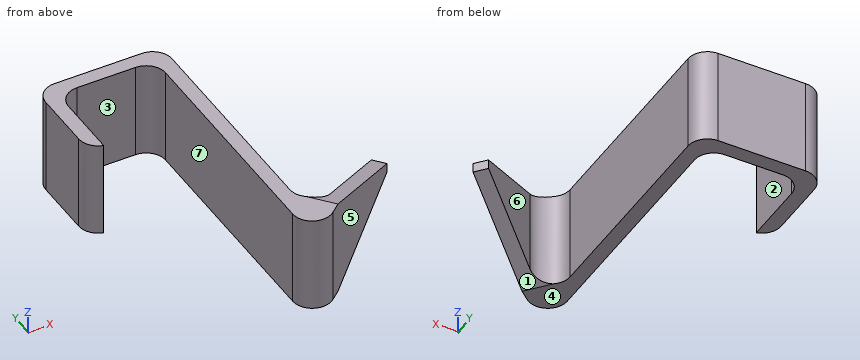
from build123d import *

# Parameters (mm, degrees)
F1_DEPTH     = 25.4
F2_T1_DEPTH  = 25.4
F2_T3_DEPTH  = 25.4
F2_T5_DEPTH  = 25.4
F2_T7_DEPTH  = 50.8
F2_T9_DEPTH  = 50.8
F2_T11_DEPTH = 49.9934442484
F3_SIZE2     = 11.4636064984
F3_SIZE      = 31.496
F3_2_SIZE2   = 11.4636064984
F3_2_SIZE    = 31.496
F4_T1_DEPTH  = 50.8
F5_T1_DEPTH  = 68.1227876391


# Not quite as in the source:
# - a fillet or chamfer that OpenCascade refuses, or shapes differently, is made with other operations: its cross-section is extruded or revolved along the edge and cut away or added


with BuildPart() as f1:
    # F0 (on Top) → F1 (new body)
    with BuildSketch(Plane.XY):
        Polygon((33.02, 0), (0, 0), (0, -25.4), (3.81, -25.4), (3.81, -3.81), (29.21, -3.81), (29.21, -76.2), (33.02, -76.2), (33.02, -71.2263982276), align=None)
        Polygon((61.7030253754, -47.1584822141), (33.02, -71.2263982276), (33.02, -76.2), (64.1520461684, -50.0771115423), align=None)
    extrude(amount=F1_DEPTH)

    # F2: fillet of radius 5.08 on 6 edges, made by hand

    # F2_s2 → F2_t1 (join)
    with BuildSketch(Plane.XY):
        with BuildLine():
            ThreePointArc((3.81, -8.89), (5.2978975516, -5.2978975516), (8.89, -3.81))
            Line((8.89, -3.81), (3.81, -3.81))
            Line((3.81, -3.81), (3.81, -8.89))
        make_face()
    extrude(amount=F2_T1_DEPTH)

    # F2_s4 → F2_t3 (join)
    with BuildSketch(Plane.XY):
        with BuildLine():
            ThreePointArc((24.13, -3.81), (27.7221024484, -5.2978975516), (29.21, -8.89))
            Line((29.21, -8.89), (29.21, -3.81))
            Line((29.21, -3.81), (24.13, -3.81))
        make_face()
    extrude(amount=F2_T3_DEPTH)

    # F2_s6 → F2_t5 (join)
    with BuildSketch(Plane.XY):
        with BuildLine():
            ThreePointArc((33.02, -60.3323030715), (35.9530992304, -64.9363466296), (41.3653610572, -64.2238088425))
            Line((41.3653610572, -64.2238088425), (33.02, -71.2263982276))
            Line((33.02, -71.2263982276), (33.02, -60.3323030715))
        make_face()
    extrude(amount=F2_T5_DEPTH)

    # F2_s8 → F2_t7 (cut)
    with BuildSketch(Plane.XY.offset(-12.7)):
        with BuildLine():
            ThreePointArc((27.94, 0), (31.5321024484, -1.4878975516), (33.02, -5.08))
            Line((33.02, -5.08), (33.02, 0))
            Line((33.02, 0), (27.94, 0))
        make_face()
    extrude(amount=F2_T7_DEPTH, mode=Mode.SUBTRACT)

    # F2_s10 → F2_t9 (cut)
    with BuildSketch(Plane.XY.offset(-12.7)):
        with BuildLine():
            ThreePointArc((5.08, 0), (1.4878975516, -1.4878975516), (0, -5.08))
            Line((0, -5.08), (0, 0))
            Line((0, 0), (5.08, 0))
        make_face()
    extrude(amount=F2_T9_DEPTH, mode=Mode.SUBTRACT)

    # F2_s12 → F2_t11 (cut)
    with BuildSketch(Plane.XY.offset(-12.2967221242)):
        with BuildLine():
            ThreePointArc((3.81, -25.4), (1.0639073716, -23.5921631237), (0, -20.4813111503))
            Line((0, -20.4813111503), (0, -25.4))
            Line((0, -25.4), (3.81, -25.4))
        make_face()
    extrude(amount=F2_T11_DEPTH, mode=Mode.SUBTRACT)

    # F3
    f3_edges = [f1.edges().sort_by_distance(p)[0] for p in [
        (62.927536, -48.617797, 25.4),
    ]]
    f3_side = f1.faces().sort_by_distance((30.827761, -2.192239, 25.4))[0]
    chamfer(f3_edges, length=F3_SIZE, length2=F3_SIZE2, reference=f3_side)

    # F3#2
    f3_2_edges = [f1.edges().sort_by_distance(p)[0] for p in [
        (62.927536, -48.617797, 0),
    ]]
    f3_2_side = f1.faces().sort_by_distance((30.827761, -2.192239, 0))[0]
    chamfer(f3_2_edges, length=F3_2_SIZE, length2=F3_2_SIZE2, reference=f3_2_side)

    # F4: fillet of radius 5.08 on 1 edges, made by hand

    # F4_s2 → F4_t1 (cut)
    with BuildSketch(Plane.XY.offset(-12.7)):
        with BuildLine():
            ThreePointArc((34.29, -76.2), (30.6978975516, -74.7121024484), (29.21, -71.12))
            Line((29.21, -71.12), (29.21, -76.2))
            Line((29.21, -76.2), (34.29, -76.2))
        make_face()
    extrude(amount=F4_T1_DEPTH, mode=Mode.SUBTRACT)

    # F5: fillet of radius 5.08 on 1 edges, made by hand

    # F5_s2 → F5_t1 (cut)
    with BuildSketch(Plane.XY.offset(-21.3613938196)):
        with BuildLine():
            ThreePointArc((37.5553610572, -72.3943802096), (32.1430992304, -73.1069179967), (29.21, -68.5028744386))
            Line((29.21, -68.5028744386), (28.702, -68.5028744386))
            ThreePointArc((28.702, -68.5028744386), (28.702, -71.12), (33.0571094194, -76.5702958467))
            Line((33.0571094194, -76.5702958467), (33.495726487, -76.4639649832))
            Line((33.495726487, -76.4639649832), (37.8818971629, -72.7835307867))
            Line((37.8818971629, -72.7835307867), (37.5553610572, -72.3943802096))
        make_face()
    extrude(amount=F5_T1_DEPTH, mode=Mode.SUBTRACT)


solid = f1.part
Design review of the part built by this model. Coordinates are the model's own, in mm. Face numbers are marked on the shaded views. A direction names the side the tool comes from. Round coordinates to 2 decimals unless told otherwise and drop trailing zeros. Order: outer loops, then holes, each group sorted by start corner. A loop starts at its lowest first (then second) coordinate and runs counter-clockwise, first axis right, second up.
1) Consider section C-C (y = -52). State the section outline as (x, z) points.
The answers:
outline: (29.21, 0) - (33.02, 0) - (33.02, 25.4) - (29.21, 25.4) - close; (55.93, 8.72) - (61.86, 10.37) - (61.86, 15.03) - (55.93, 16.68) - close
2) For L1, parallel to X at y = -20, z = 23.25; L2, parallel to X at y = -31, z = 5.5; L3, parallel to Y at x = 23, z = 15, list the stretches that pass through material, from the lowest coordinate up.
The answers:
L1: x = 0 to 3.81, 29.21 to 33.02
L2: x = 29.21 to 33.02
L3: y = -3.81 to 0
3) Machinability: for the marked faces 5, 6 and 7, which of the approach directions +Z, -Z, +X, -X, +Y, -Y give a long, thin tool a straight path to every point of the face, cutting with its end or side? Answer none if there is none.
The answers:
face 5: +Z, -Z, +X, -Y
face 6: +Z, -Z, +Y
face 7: +Z, -Z, -Y
4) Draft analysis for pull direction X (two halves, no side actions). For the marked faces 1, 2, 3 and 4, state which applies: released by +X, released by -X, zero draft, split by the parting line, or undercut.
The answers:
face 1: released by +X
face 2: undercut
face 3: undercut
face 4: zero draft
5) Clearance check with flat-ended pins moving along their axes: pin 1 Ø7.5 at (x, z) = (19, 15) entering from -Y; pin 2 Ø5 at (x, y) = (33.5, -39.5) entering from -Z; pin 3 Ø5 at (y, z) = (-57, 7) entering from +X; pin 4 Ø12.5 at (y, z) = (-41, 18) entering from -X. State where each tip first meets the part, or that it passes through.
The answers:
pin 1: stops at y = -3.81
pin 2: stops at z = 0
pin 3: stops at x = 58.17
pin 4: stops at x = 29.21
6) Consider section A-A (y = -12). State the section outline as (x, z) points.
The answers:
outline: (0, 0) - (3.81, 0) - (3.81, 25.4) - (0, 25.4) - close; (29.21, 0) - (33.02, 0) - (33.02, 25.4) - (29.21, 25.4) - close
7) Consider section D-D (x = 31). State the section outline as (y, z) points, plus the area to 3 significant figures.
The answers:
outline: (-72.37, 0) - (-1.03, 0) - (-1.03, 25.4) - (-72.37, 25.4) - close
area: 1,810 mm2
8) Consider section B-B (z = 3.5). State the section outline as (x, y) points, plus the area to 3 significant figures.
The answers:
outline: (0, -20.48) arc R5.08 ccw to (3.81, -25.4) - (3.81, -8.89) arc R5.08 cw to (8.89, -3.81) - (24.13, -3.81) arc R5.08 cw to (29.21, -8.89) - (29.21, -68.5) arc R5.08 ccw to (37.56, -72.39) - (47.39, -64.14) - (44.94, -61.22) - (41.37, -64.22) arc R5.08 cw to (33.02, -60.33) - (33.02, -5.08) arc R5.08 ccw to (27.94, 0) - (5.08, 0) arc R5.08 ccw to (0, -5.08) - close
area: 550 mm2
